from build123d import *

# Parameters (mm, degrees)
BOSS_EXTRUDE1_DEPTH = 34
SKETCH3_R           = 35
CUT_EXTRUDE1_DEPTH  = 18
CUT_EXTRUDE2_DEPTH  = 20


with BuildPart() as part:
    # Sketch1 → Boss-Extrude1 (new body)
    with BuildSketch(Plane.XY):
        with BuildLine():
            Line((75, 40), (0, 40))
            ThreePointArc((0, 40), (-40, 0), (0, -40))
            Line((0, -40), (75, -40))
            Line((75, -40), (75, -22))
            ThreePointArc((75, -22), (53, 0), (75, 22))
            Line((75, 22), (75, 40))
        make_face()
    extrude(amount=BOSS_EXTRUDE1_DEPTH)

    # Sketch3 → Cut-Extrude1 (cut)
    with BuildSketch(Plane.XY.offset(34)):
        with Locations((10, 0)):
            Circle(SKETCH3_R)
    extrude(amount=-CUT_EXTRUDE1_DEPTH, mode=Mode.SUBTRACT)

    # Sketch4 → Cut-Extrude2 (cut)
    with BuildSketch(Plane.XY.offset(34)):
        with BuildLine():
            ThreePointArc((53.833989511, -6), (53, 0), (53.833989511, 6))
            Line((53.833989511, 6), (44.481879299, 6))
            Line((44.481879299, 6), (16, 6))
            Line((16, 6), (16, 34.481879299))
            Line((16, 34.481879299), (16, 40))
            Line((16, 40), (4, 40))
            Line((4, 40), (4, 34.481879299))
            Line((4, 34.481879299), (4, 6))
            Line((4, 6), (-24.481879299, 6))
            Line((-24.481879299, 6), (-39.547439867, 6))
            ThreePointArc((-39.547439867, 6), (-40, 0), (-39.547439867, -6))
            Line((-39.547439867, -6), (-24.481879299, -6))
            Line((-24.481879299, -6), (4, -6))
            Line((4, -6), (4, -34.481879299))
            Line((4, -34.481879299), (4, -40))
            Line((4, -40), (16, -40))
            Line((16, -40), (16, -34.481879299))
            Line((16, -34.481879299), (16, -6))
            Line((16, -6), (44.481879299, -6))
            Line((44.481879299, -6), (53.833989511, -6))
        make_face()
    extrude(amount=-CUT_EXTRUDE2_DEPTH, mode=Mode.SUBTRACT)


solid = part.part
Design review of the part built by this model. Coordinates are the model's own, in mm. A direction names the side the tool comes from. Round coordinates to 2 decimals unless told otherwise and drop trailing zeros. Loops run counter-clockwise (first coordinate to the right, second up) from the corner with the lowest first, then second, coordinate; pieces in that order, holes last. Notation, with made-up numbers: M 44.5,-0.75 L 100.5,-0.75 A25 cw 100.5,14.25 Z; hole C 75,-37 d6. An arc over 180 degrees is marked long. Answer as a JSON object with one key per item and string values.
Item 1: We need section D-D on x = 41. Give the boundary of the cut face in (y, z), and give its area (3 significant figures).
Answer sheet:
{"outline": "M -40,0 L 40,0 L 40,34 L 16.25,34 L 16.25,16 L 6,16 L 6,14 L -6,14 L -6,16 L -16.25,16 L -16.25,34 L -40,34 Z", "area": "2,110 mm^2"}
Item 2: Machinability: for faces 4 (the flat face through (45, 6, 22)), 5 (the flat face through (4, 36, 21)), 6 (the flat face through (-7, 17, 16)), which of the approach directions +Z, -Z, +X, -X, +Y, -Y give a long, thin tool a straight path to every point of the face, cutting with its end or side? Answer none if there is none.
Answer sheet:
{"face 4": "+Z, +X, -X", "face 5": "+Z, +Y, -Y", "face 6": "+Z"}
Item 3: We need section A-A on z = 26.5. Give the boundary of the cut face in (x, y).
Answer sheet:
{"outline": "M -39.55,-6 A40 ccw 0,-40 L 4,-40 L 4,-34.48 A35 cw -24.48,-6 Z; M -39.55,6 L -24.48,6 A35 cw 4,34.48 L 4,40 L 0,40 A40 ccw Z; M 16,-40 L 75,-40 L 75,-22 A22 cw 53.83,-6 L 44.48,-6 A35 cw 16,-34.48 Z; M 16,34.48 A35 cw 44.48,6 L 53.83,6 A22 cw 75,22 L 75,40 L 16,40 Z"}
Item 4: The part is to be moulded in two halves that separate along Y. For faces 1 (the flat face through (38, 40, 17)), 2 (the flat face through (4, -36, 20)), 3 (the cylindrical face through (-14.96, -24.535, 25.126)), say which applies: pulls with the +Y half, pulls with the -Y half, needs draft (parallel to the pull), parting line crosses it, or undercut.
Answer sheet:
{"face 1": "pulls with the +Y half", "face 2": "needs draft", "face 3": "undercut"}
Item 5: We need section B-B on x = 66. Give the boundary of the cut face in (y, z), and give its area (3 significant figures).
Answer sheet:
{"outline": "M -40,0 L -20.07,0 L -20.07,34 L -40,34 Z; M 20.07,0 L 40,0 L 40,34 L 20.07,34 Z", "area": "1,350 mm^2"}
Item 6: Wall thickness on L1, parallel to Z at x = 7.5, y = 25; L2, parallel to Y at x = 19.5, z = 21; L3, parallel to X at y = -27, z = 15.5: over which ranges is each line inside the solid? List them lowest first. Write a range as from..to.
Answer sheet:
{"L1": "z = 0..14", "L2": "y = -40..-33.69, 33.69..40", "L3": "x = -29.51..4, 16..75"}
Item 7: Clearance check with flat-ended pins moving along their axes: P1, Ø10, axis at y = 14.5, z = 21, coming from the -X side; P2, Ø6, axis at y = 17, z = 20.5, coming from the +X side; P3, Ø1, axis at x = -19.5, z = 6.5, coming from the -Y side. State where each tip first meets the part, or that it passes through.
Answer sheet:
{"P1": "stops at x = -38.86", "P2": "stops at x = 65.83", "P3": "stops at y = -35.2"}
Item 8: We need section C-C on y = 0. Give the boundary of the cut face in (x, z), and give its area (3 significant figures).
Answer sheet:
{"outline": "M -40,0 L 53,0 L 53,14 L -40,14 Z", "area": "1,300 mm^2"}
